from build123d import *

# Parameters (mm, degrees)
BOSS_EXTRUDE2_DEPTH = 10
SKETCH3_W           = 29.532068245
SKETCH3_H           = 5.332178988
SKETCH3_W_2         = 29.737152051
SKETCH3_W_3         = 30.967654895
SKETCH3_W_4         = 26.86597875
BOSS_EXTRUDE3_DEPTH = 0.5
SCALE1_SCALE        = 5


with BuildPart() as part:
    # Sketch2 → Boss-Extrude2 (new body)
    with BuildSketch(Plane.XY):
        Polygon((0, 0), (16.944463815, 48.421938639), (198.277369744, 50.219093306), (181.332905929, 1.797154667), align=None)
    extrude(amount=BOSS_EXTRUDE2_DEPTH)

    # Sketch3 → Boss-Extrude3 (add)
    with BuildSketch(Plane(origin=(0, 0, 0), x_dir=(-1, 0, 0), z_dir=(0, 0, -1))):
        with Locations((-160.253659434, 25.929881882)):
            Rectangle(SKETCH3_W, SKETCH3_H)
        with Locations((-113.802177091, 26.134965689)):
            Rectangle(SKETCH3_W_2, SKETCH3_H)
        with Locations((-67.453236652, 25.929881882)):
            Rectangle(SKETCH3_W_3, SKETCH3_H)
        with Locations((-29.51273231, 26.134965689)):
            Rectangle(SKETCH3_W_4, SKETCH3_H)
    extrude(amount=BOSS_EXTRUDE3_DEPTH)


with BuildPart() as part_1:
    # Scale1: scaled about (99.120137523, 25.112815696, 4.981334283)
    add(part.part.scale(SCALE1_SCALE).moved(Location((-396.480550092, -100.451262784, -19.925337132))))


solid = part_1.part
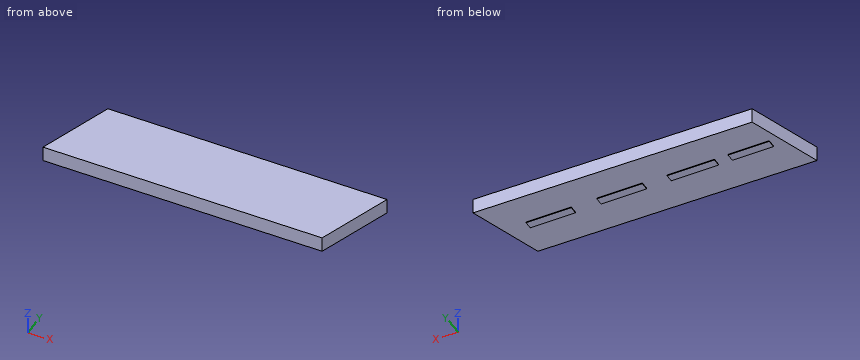
For this review, take the finished solid that the model builds, in its own axes (mm). Round coordinates to 2 decimals unless told otherwise and drop trailing zeros. Order: outer loops, then holes, each group sorted by start corner. A loop starts at its lowest first (then second) coordinate and runs counter-clockwise, first axis right, second up. Notation, with made-up numbers: M -34,-6 L 22,-6 A26 cw 22,33 Z; hole C 66,7.5 d4. An arc over 180 degrees is marked long. Use a Markdown table: item, result. Add a question column.
Item 1: To check wall thickness, follow line 1 along Z through (x, y) = (-161.5, 56.5); line 2 along Y through (x, z) = (173.5, 12); line 3 along Y through (x, z) = (-244, 26). State the ranges of each line that lie inside material, in increasing order.
Item 2: Insertion check: pin 1 (1.2 mm diameter, centred on x = -271, z = -21.5, fed in from -Y); pin 2 (1 mm diameter, centred on y = 124.5, z = 7.5, fed in from +X); pin 3 (3 mm diameter, centred on y = 31.5, z = -21, fed in from -X). Each pin has a flat end and moves straight along its axis. Give the tip position at first contact, or say it passes through.
Item 3: Add section B-B, the plane y = -32. Give the boundary of the cut face in (x, z), then the cut area to 3 significant figures.
Item 4: Add section A-A, the plane x = 363. Give the boundary of the cut face in (y, z), then the cut area to 3 significant figures.
Item 5: Add section C-C, the plane z = 14. Give the boundary of the cut face in (x, y), then the cut area to 3 significant figures.
Geometry results:
| question | item | result |
|---|---|---|
| 1 | line 1 | z = -19.93 to 30.07 |
| 1 | line 2 | y = -94.8 to 146.47 |
| 1 | line 3 | y = -98.94 to 142.33 |
| 2 | pin 1 | stops at y = 16.89 |
| 2 | pin 2 | stops at x = 585.93 |
| 2 | pin 3 | stops at x = -350.67 |
| 3 | outline | M -372.53,-19.93 L 530.99,-19.93 L 530.99,30.07 L -372.53,30.07 Z |
| 3 | area | 45,200 mm² |
| 4 | outline | M -92.92,-19.93 L 15.87,-19.93 L 15.87,-22.43 L 42.53,-22.43 L 42.53,-19.93 L 148.35,-19.93 L 148.35,30.07 L -92.92,30.07 Z |
| 4 | area | 12,100 mm² |
| 5 | outline | M -396.48,-100.45 L 510.18,-91.47 L 594.91,150.64 L -311.76,141.66 Z |
| 5 | area | 219,000 mm² |
